```python
from build123d import *

# Parameters (mm, degrees)
BOSS_EXTRUDE1_DEPTH = 6.35
SKETCH2_R           = 1.905
CUT_EXTRUDE1_DEPTH  = 6.35
CHAMFER1_SIZE       = 6.35
FILLET2_R           = 1.5875


with BuildPart() as part:
    # Sketch1 → Boss-Extrude1 (new body)
    with BuildSketch(Plane(origin=(0, 0, 0), x_dir=(1, 0, 0), z_dir=(0, 1, 0))):
        Polygon((-33.3375, 0), (33.3375, 0), (33.3375, 36.6395), (23.8125, 36.6395), (23.8125, 6.35), (-23.8125, 6.35), (-23.8125, 36.6395), (-33.3375, 36.6395), align=None)
    extrude(amount=BOSS_EXTRUDE1_DEPTH)

    # Sketch2 → Cut-Extrude1 (cut)
    with BuildSketch(Plane(origin=(0, 0, -36.6395), x_dir=(-1, 0, 0), z_dir=(0, 0, -1))):
        with Locations((-28.575, 3.175)):
            Circle(SKETCH2_R)
    cut_extrude1 = extrude(amount=-CUT_EXTRUDE1_DEPTH, mode=Mode.SUBTRACT)

    # Mirror1: Cut-Extrude1 across plane
    add(cut_extrude1.mirror(Plane(origin=(0, 0, 0), x_dir=(0, 0, 1), z_dir=(1, 0, 0))), mode=Mode.SUBTRACT)

    # Chamfer1
    chamfer1_edges = [part.edges().sort_by_distance(p)[0] for p in [
        (33.3375, 3.175, 0),
        (-33.3375, 3.175, 0),
    ]]
    chamfer(chamfer1_edges, length=CHAMFER1_SIZE)

    # Fillet2
    # the kernel refuses this fillet: 1.5875 mm, written as the material it adds along each edge
    with BuildSketch(Plane(origin=(-23.8125, 0, -6.35), x_dir=(0, 0, -1), z_dir=(0, 1, 0))) as fillet2_piece_1:
        with BuildLine():
            CenterArc((FILLET2_R, -FILLET2_R), FILLET2_R, 90, 90)
            Line((0, -FILLET2_R), (0, 0))
            Line((0, 0), (FILLET2_R, 0))
        make_face()
    extrude(amount=6.35)
    with BuildSketch(Plane(origin=(23.8125, 0, -6.35), x_dir=(0, 0, -1), z_dir=(0, 1, 0))) as fillet2_piece_2:
        with BuildLine():
            CenterArc((FILLET2_R, FILLET2_R), FILLET2_R, 180, 90)
            Line((0, FILLET2_R), (0, 0))
            Line((0, 0), (FILLET2_R, 0))
        make_face()
    extrude(amount=6.35)
    # the kernel refuses this fillet: 1.5875 mm, written as the material it takes off along each edge
    with BuildSketch(Plane(origin=(-31.75, 4.7625, -35.052), x_dir=(-1, 0, 0), z_dir=(0, 1, 0))) as fillet2_2_piece_1_section:
        Polygon((0, 0), (FILLET2_R, 0), (FILLET2_R, -FILLET2_R), (0, -FILLET2_R), align=None)
    fillet2_2_piece_1 = extrude(amount=FILLET2_R, mode=Mode.PRIVATE)
    fillet2_2_piece_1 = fillet2_2_piece_1 - Plane(origin=(-31.75, 4.7625, -35.052), x_dir=(0.7071067811865475, 0, 0.7071067811865475), z_dir=(0, 1, 0)) * Sphere(FILLET2_R, mode=Mode.PRIVATE)
    add(fillet2_2_piece_1, mode=Mode.SUBTRACT)
    with BuildSketch(Plane(origin=(31.75, 4.7625, -35.052), x_dir=(0, 1, 0), z_dir=(0, 0, -1))) as fillet2_2_piece_2_section:
        Polygon((0, 0), (FILLET2_R, 0), (FILLET2_R, FILLET2_R), (0, FILLET2_R), align=None)
    fillet2_2_piece_2 = extrude(amount=FILLET2_R, mode=Mode.PRIVATE)
    fillet2_2_piece_2 = fillet2_2_piece_2 - Plane(origin=(31.75, 4.7625, -35.052), x_dir=(-0.7071067811865475, -0.7071067811865475, 0), z_dir=(0, 0, -1)) * Sphere(FILLET2_R, mode=Mode.PRIVATE)
    add(fillet2_2_piece_2, mode=Mode.SUBTRACT)
    with BuildSketch(Plane(origin=(-26.32993597, 4.7625, -1.5875), x_dir=(0, 0, 1), z_dir=(0, 1, 0))) as fillet2_2_piece_3_section:
        Polygon((0, 0), (FILLET2_R, 0), (FILLET2_R, -FILLET2_R * 0.414213562373), (FILLET2_R * 0.707106781187, -FILLET2_R * 0.707106781187), align=None)
    fillet2_2_piece_3 = extrude(amount=FILLET2_R, mode=Mode.PRIVATE)
    fillet2_2_piece_3 = fillet2_2_piece_3 - Plane(origin=(-26.32993597, 4.7625, -1.5875), x_dir=(0.38268343236508956, 0, -0.9238795325112867), z_dir=(0, 1, 0)) * Sphere(FILLET2_R, mode=Mode.PRIVATE)
    add(fillet2_2_piece_3, mode=Mode.SUBTRACT)
    with BuildSketch(Plane(origin=(26.32993597, 4.7625, -1.5875), x_dir=(0, 0, 1), z_dir=(0, 1, 0))) as fillet2_2_piece_4_section:
        Polygon((0, 0), (FILLET2_R, 0), (FILLET2_R, FILLET2_R * 0.414213562373), (FILLET2_R * 0.707106781187, FILLET2_R * 0.707106781187), align=None)
    fillet2_2_piece_4 = extrude(amount=FILLET2_R, mode=Mode.PRIVATE)
    fillet2_2_piece_4 = fillet2_2_piece_4 - Plane(origin=(26.32993597, 4.7625, -1.5875), x_dir=(-0.3826834323650899, 0, -0.9238795325112866), z_dir=(0, 1, 0)) * Sphere(FILLET2_R, mode=Mode.PRIVATE)
    add(fillet2_2_piece_4, mode=Mode.SUBTRACT)
    with BuildSketch(Plane(origin=(-31.75, 4.7625, -7.00756403), x_dir=(-1, 0, 0), z_dir=(0, 1, 0))) as fillet2_2_piece_5_section:
        Polygon((0, 0), (FILLET2_R, 0), (FILLET2_R, FILLET2_R * 0.414213562373), (FILLET2_R * 0.707106781187, FILLET2_R * 0.707106781187), align=None)
    fillet2_2_piece_5 = extrude(amount=FILLET2_R, mode=Mode.PRIVATE)
    fillet2_2_piece_5 = fillet2_2_piece_5 - Plane(origin=(-31.75, 4.7625, -7.00756403), x_dir=(0.9238795325112866, 0, -0.38268343236508984), z_dir=(0, 1, 0)) * Sphere(FILLET2_R, mode=Mode.PRIVATE)
    add(fillet2_2_piece_5, mode=Mode.SUBTRACT)
    with BuildSketch(Plane(origin=(31.75, 4.7625, -7.00756403), x_dir=(1, 0, 0), z_dir=(0, 1, 0))) as fillet2_2_piece_6_section:
        Polygon((0, 0), (FILLET2_R, 0), (FILLET2_R, -FILLET2_R * 0.414213562373), (FILLET2_R * 0.707106781187, -FILLET2_R * 0.707106781187), align=None)
    fillet2_2_piece_6 = extrude(amount=FILLET2_R, mode=Mode.PRIVATE)
    fillet2_2_piece_6 = fillet2_2_piece_6 - Plane(origin=(31.75, 4.7625, -7.00756403), x_dir=(-0.9238795325112868, 0, -0.38268343236508967), z_dir=(0, 1, 0)) * Sphere(FILLET2_R, mode=Mode.PRIVATE)
    add(fillet2_2_piece_6, mode=Mode.SUBTRACT)
    with BuildSketch(Plane(origin=(-33.3375, -3.96875, -36.6395), x_dir=(0, 0, 1), z_dir=(0, 1, 0))) as fillet2_2_piece_7:
        with BuildLine():
            CenterArc((FILLET2_R, FILLET2_R), FILLET2_R, 180, 90)
            Line((0, FILLET2_R), (0, 0))
            Line((0, 0), (FILLET2_R, 0))
        make_face()
    extrude(amount=8.73125, mode=Mode.SUBTRACT)
    with BuildSketch(Plane(origin=(-23.8125, -3.96875, -36.6395), x_dir=(-1, 0, 0), z_dir=(0, 1, 0))) as fillet2_2_piece_8:
        with BuildLine():
            CenterArc((FILLET2_R, FILLET2_R), FILLET2_R, 180, 90)
            Line((0, FILLET2_R), (0, 0))
            Line((0, 0), (FILLET2_R, 0))
        make_face()
    extrude(amount=14.2875, mode=Mode.SUBTRACT)
    with BuildSketch(Plane(origin=(23.8125, -3.96875, -36.6395), x_dir=(1, 0, 0), z_dir=(0, 1, 0))) as fillet2_2_piece_9:
        with BuildLine():
            CenterArc((FILLET2_R, -FILLET2_R), FILLET2_R, 90, 90)
            Line((0, -FILLET2_R), (0, 0))
            Line((0, 0), (FILLET2_R, 0))
        make_face()
    extrude(amount=14.2875, mode=Mode.SUBTRACT)
    with BuildSketch(Plane(origin=(33.3375, -3.96875, -36.6395), x_dir=(0, 0, 1), z_dir=(0, 1, 0))) as fillet2_2_piece_10:
        with BuildLine():
            CenterArc((FILLET2_R, -FILLET2_R), FILLET2_R, 90, 90)
            Line((0, -FILLET2_R), (0, 0))
            Line((0, 0), (FILLET2_R, 0))
        make_face()
    extrude(amount=8.73125, mode=Mode.SUBTRACT)
    with BuildSketch(Plane(origin=(31.75, 6.35, -36.6395), x_dir=(0, 0, 1), z_dir=(-1, 0, 0)), Plane(origin=(-19.84375, 6.35, -36.6395), x_dir=(0, 0, 1), z_dir=(-1, 0, 0))) as fillet2_2_piece_11:
        with BuildLine():
            CenterArc((FILLET2_R, -FILLET2_R), FILLET2_R, 90, 90)
            Line((0, -FILLET2_R), (0, 0))
            Line((0, 0), (FILLET2_R, 0))
        make_face()
    extrude(amount=11.90625, mode=Mode.SUBTRACT)
    with BuildSketch(Plane(origin=(-26.32993597, 6.35, 0), x_dir=(0, -1, 0), z_dir=(1, 0, 0))) as fillet2_2_piece_12:
        with BuildLine():
            CenterArc((FILLET2_R, FILLET2_R), FILLET2_R, 180, 90)
            Line((0, FILLET2_R), (0, 0))
            Line((0, 0), (FILLET2_R, 0))
        make_face()
    extrude(amount=52.659871939, mode=Mode.SUBTRACT)
    with BuildSketch(Plane(origin=(26.9875, -1.643910076, 0), x_dir=(-1, 0, 0), z_dir=(0, 1, 0)), Plane(origin=(33.3375, -1.643910076, -6.35), x_dir=(-0.7071067811865448, 0, 0.7071067811865502), z_dir=(0, 1, 0))) as fillet2_2_piece_13:
        with BuildLine():
            CenterArc((FILLET2_R * 0.414213562373, -FILLET2_R), FILLET2_R, 90, 45)
            Line((-FILLET2_R * 0.292893218813, -FILLET2_R * 0.292893218813), (0, 0))
            Line((0, 0), (FILLET2_R * 0.414213562373, 0))
        make_face()
    extrude(amount=6.406410076, mode=Mode.SUBTRACT)
    with BuildSketch(Plane(origin=(-26.9875, -1.643910076, 0), x_dir=(1, 0, 0), z_dir=(0, 1, 0)), Plane(origin=(-33.3375, -1.643910076, -6.35), x_dir=(0.7071067811865468, 0, 0.7071067811865482), z_dir=(0, 1, 0))) as fillet2_2_piece_14:
        with BuildLine():
            CenterArc((FILLET2_R * 0.414213562373, FILLET2_R), FILLET2_R, 225, 45)
            Line((-FILLET2_R * 0.292893218813, FILLET2_R * 0.292893218813), (0, 0))
            Line((0, 0), (FILLET2_R * 0.414213562373, 0))
        make_face()
    extrude(amount=6.406410076, mode=Mode.SUBTRACT)
    with BuildSketch(Plane(origin=(33.3375, 6.35, -7.00756403), x_dir=(-1, 0, 0), z_dir=(0, 0, -1)), Plane(origin=(-33.3375, 6.35, -35.052), x_dir=(1, 0, 0), z_dir=(0, 0, 1))) as fillet2_2_piece_15:
        with BuildLine():
            CenterArc((FILLET2_R, -FILLET2_R), FILLET2_R, 90, 90)
            Line((0, -FILLET2_R), (0, 0))
            Line((0, 0), (FILLET2_R, 0))
        make_face()
    extrude(amount=28.04443597, mode=Mode.SUBTRACT)
    with BuildSketch(Plane(origin=(27.452467985, 6.35, -0.464967985), x_dir=(0, -1, 0), z_dir=(0.7071067811865476, 0, -0.7071067811865476))) as fillet2_2_piece_16:
        with BuildLine():
            CenterArc((FILLET2_R, FILLET2_R), FILLET2_R, 180, 90)
            Line((0, FILLET2_R), (0, 0))
            Line((0, 0), (FILLET2_R, 0))
        make_face()
    extrude(amount=7.665128061, mode=Mode.SUBTRACT)
    with BuildSketch(Plane(origin=(-27.452467985, 6.35, -0.464967985), x_dir=(0, -1, 0), z_dir=(-0.7071067811865477, 0, -0.7071067811865475))) as fillet2_2_piece_17:
        with BuildLine():
            CenterArc((FILLET2_R, -FILLET2_R), FILLET2_R, 90, 90)
            Line((0, -FILLET2_R), (0, 0))
            Line((0, 0), (FILLET2_R, 0))
        make_face()
    extrude(amount=7.665128061, mode=Mode.SUBTRACT)
    # the kernel refuses this fillet: 1.5875 mm, written as the material it takes off along each edge
    with BuildSketch(Plane(origin=(-25.4, 4.7625, -35.052), x_dir=(0, 1, 0), z_dir=(1, 0, 0))) as fillet2_3_piece_1_section:
        Polygon((0, 0), (FILLET2_R, 0), (FILLET2_R, -FILLET2_R), (0, -FILLET2_R), align=None)
    fillet2_3_piece_1 = extrude(amount=FILLET2_R, mode=Mode.PRIVATE)
    fillet2_3_piece_1 = fillet2_3_piece_1 - Plane(origin=(-25.4, 4.7625, -35.052), x_dir=(0, -0.7071067811865475, 0.7071067811865475), z_dir=(1, 0, 0)) * Sphere(FILLET2_R, mode=Mode.PRIVATE)
    add(fillet2_3_piece_1, mode=Mode.SUBTRACT)
    with BuildSketch(Plane(origin=(25.4, 4.7625, -35.052), x_dir=(0, 1, 0), z_dir=(-1, 0, 0))) as fillet2_3_piece_2_section:
        Polygon((0, 0), (FILLET2_R, 0), (FILLET2_R, FILLET2_R), (0, FILLET2_R), align=None)
    fillet2_3_piece_2 = extrude(amount=FILLET2_R, mode=Mode.PRIVATE)
    fillet2_3_piece_2 = fillet2_3_piece_2 - Plane(origin=(25.4, 4.7625, -35.052), x_dir=(0, -0.7071067811865475, 0.7071067811865475), z_dir=(-1, 0, 0)) * Sphere(FILLET2_R, mode=Mode.PRIVATE)
    add(fillet2_3_piece_2, mode=Mode.SUBTRACT)
    with BuildSketch(Plane(origin=(23.8125, 6.35, -35.052), x_dir=(0, -1, 0), z_dir=(0, 0, 1)), Plane(origin=(-23.8125, 6.35, -7.9375), x_dir=(0, -1, 0), z_dir=(0, 0, -1))) as fillet2_3_piece_3:
        with BuildLine():
            CenterArc((FILLET2_R, FILLET2_R), FILLET2_R, 180, 90)
            Line((0, FILLET2_R), (0, 0))
            Line((0, 0), (FILLET2_R, 0))
        make_face()
    extrude(amount=27.1145, mode=Mode.SUBTRACT)
    with BuildSketch(Plane(origin=(22.225, 6.35, -6.35), x_dir=(0, -1, 0), z_dir=(-1, 0, 0))) as fillet2_3_piece_4:
        with BuildLine():
            CenterArc((FILLET2_R, FILLET2_R), FILLET2_R, 180, 90)
            Line((0, FILLET2_R), (0, 0))
            Line((0, 0), (FILLET2_R, 0))
        make_face()
    extrude(amount=44.45, mode=Mode.SUBTRACT)
    with BuildSketch(Plane(origin=(-22.225, 6.35, -7.9375), x_dir=(-1, 0, 0), z_dir=(0, 0, -1))) as fillet2_3_piece_5:
        with BuildLine():
            CenterArc((1.5875 + FILLET2_R, -FILLET2_R), FILLET2_R, 90, 90)
            Line((1.5875 + FILLET2_R, 0), (1.5875, 0))
            Line((1.5875, 0), (1.5875, -FILLET2_R))
        make_face()
    revolve(axis=Axis((-22.225, 6.35, -7.9375), (0, 1, 0)), revolution_arc=90, mode=Mode.SUBTRACT)
    with BuildSketch(Plane(origin=(22.225, 6.35, -7.9375), x_dir=(1, 0, 0), z_dir=(0, 0, -1))) as fillet2_3_piece_6:
        with BuildLine():
            CenterArc((1.5875 + FILLET2_R, FILLET2_R), FILLET2_R, 180, 90)
            Line((1.5875 + FILLET2_R, 0), (1.5875, 0))
            Line((1.5875, 0), (1.5875, FILLET2_R))
        make_face()
    revolve(axis=Axis((22.225, 6.35, -7.9375), (0, -1, 0)), revolution_arc=90, mode=Mode.SUBTRACT)


solid = part.part
```
Geometry: final body of the model. Coordinates: model frame, mm. A direction names the side the tool comes from. Round coordinates to 2 decimals unless told otherwise and drop trailing zeros. Use one line per item in the form item = value. Start each with the question number.
1) First-contact query: P1, Ø1.1, axis at x = 28, y = 4, coming from the -Z side. Flat tip, straight axial feed; report the tip coordinate or a pass-through.
2) Section C-C on z = -31. Give the number of separate pieces and of enclosed holes in the cut face, then the cut area to 3 significant figures.
3) Line query: L1, parallel to X at y = 2.5, z = -13.5; L2, parallel to Z at x = 4, y = 3.75; L3, parallel to X at y = 5.75, z = -21. Output: solid intervals per line, ascending.
4) Access query for faces 1 (the cylindrical face through (26.76, 3.75, -33.51)), 2 (the flat face through (33.338, 2, -21)), 3 (the cylindrical face through (24.29, 5.9, -21.68)), 4 (the flat face through (23.812, 2, -22)). Directions: +Z, -Z, +X, -X, +Y, -Y. A direction counts if a zero-diameter tool reaches every point of the face in a straight line with its end or side. Return the directions, or none.
Response:
q1.P1 = -30.29
q2.separate_pieces = 2
q2.enclosed_holes = 2
q2.area = 96.0 mm^2
q3.L1 = -33.34 to -23.81, 23.81 to 33.34
q3.L2 = -6.35 to 0
q3.L3 = -32.99 to -24.16, 24.16 to 32.99
q4.face_1 = -Z
q4.face_2 = +Z, -Z, +X, +Y, -Y
q4.face_3 = -Z, +Y
q4.face_4 = -Z, +Y, -Y
